Read the model definition and answer for the solid it produces. Units are mm, in the model's axes. Face numbers are marked on the shaded views. A direction names the side the tool comes from. Give positions to 0.01 mm unless a question says otherwise; leave off trailing zeros. One line per item, written item: value.
from build123d import *

# Parameters (mm, degrees)
F4_R          = 3.4529620344
F5_DEPTH      = 6.35
F6_W          = 3.175
F6_H          = 2.794
F7_DEPTH      = 25.4
F7_DEPTH_BACK = 12.7
F9_R          = 0.635
F10_DEPTH     = 6.35


with BuildPart() as f3:
    # F1 (on Front) → F3 section 0
    with BuildSketch(Plane.XZ):
        Polygon((12.6337242704, 3.302), (0, 4.5977665918), (-12.6337242704, 3.302), (-12.6337242704, 0), (-12.6337242704, -3.302), (0, -4.5977665918), (12.6337242704, -3.302), (12.6337242704, 0), align=None)
    # F2 (on offset) → F3 section 1
    with BuildSketch(Plane.XZ.offset(38.1)):
        Polygon((12.6239405945, -1.3549544383), (12.6239405945, 0), (12.6239405945, 1.3549544383), (0, 2.2075881716), (-12.6239405945, 1.3549544383), (-12.6239405945, 0), (-12.6239405945, -1.3549544383), (0, -2.2075881716), align=None)
    loft()

    # F4 (on Front) → F5 (join)
    with BuildSketch(Plane.XZ):
        Circle(F4_R)
    extrude(amount=-F5_DEPTH)

    # F6 (on Front) → F7 (cut, two sides)
    with BuildSketch(Plane.XZ) as f7_sk:
        Rectangle(F6_W, F6_H)
    extrude(amount=-F7_DEPTH, mode=Mode.SUBTRACT)
    extrude(f7_sk.sketch, amount=F7_DEPTH_BACK, mode=Mode.SUBTRACT)

    # F9 (on offset) → F10 (cut)
    with BuildSketch(Plane.XY.offset(6.35)):
        with Locations((0, 3.2384919468)):
            Circle(F9_R)
    extrude(amount=-F10_DEPTH, mode=Mode.SUBTRACT)


solid = f3.part
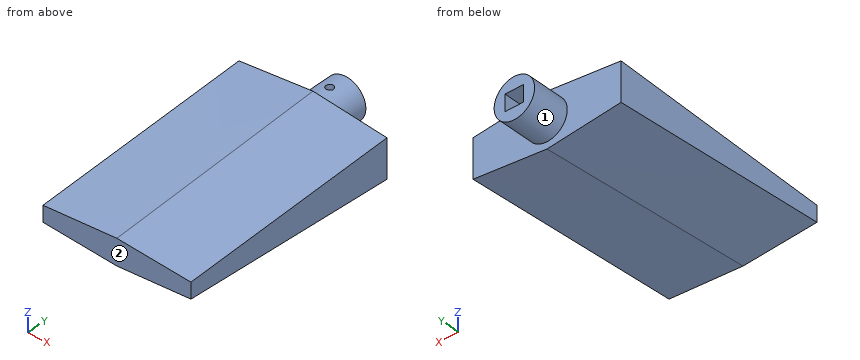
1) Consider probe 1 along X at (y, z) = (-1, 0.5); probe 2 along X at (y, z) = (-20, 0.75); probe 3 along Y at (x, z) = (3.75, 0.75). Determine where each line is inside the solid, lowest interval first.
Reported:
probe 1: x = -12.63 to -1.59, 1.59 to 12.63
probe 2: x = -12.63 to 12.63
probe 3: y = -38.1 to 0
2) Each of these flat-tipped pins is pushed along its axis until it touches: pin 1 Ø1 at (x, y) = (0, 3.24) entering from +Z; pin 2 Ø6 at (x, y) = (-4.5, 0.5) entering from -Z; pin 3 Ø1 at (x, y) = (-6, -1.5) entering from +Z. Where does it stop, or does it pass through?
Reported:
pin 1: stops at z = -1.4
pin 2: stops at z = -4.44
pin 3: stops at z = 3.95
3) Which of the six approach directions +Z, -Z, +X, -X, +Y, -Y give full straight-line access (tool end or side, diameter ignored) to the marked faces 1 and 2?
Reported:
face 1: +Y
face 2: +Z, -Z, +X, -X, -Y
